Input: part model. Units: mm. Frame: model coordinates. A direction names the side the tool comes from. Give positions to 0.01 mm unless a question says otherwise; leave off trailing zeros. Loops run counter-clockwise (first coordinate to the right, second up) from the corner with the lowest first, then second, coordinate; pieces in that order, holes last. Notation, with made-up numbers: M 8.25,-18.5 L 44.25,-18.5 A6 cw 44.25,-12.5 Z; hole C 7.25,16.25 d2. An arc over 180 degrees is marked long. Use a Markdown table: item, result. Add a question column.
Autodesk Inventor part; units mm, degrees
ref_plane "YZ Plane" through (0, 0, 0) normal (1, 0, 0) x (0, 1, 0)
ref_plane "XZ Plane" through (0, 0, 0) normal (0, 1, 0) x (-1, 0, 0)
ref_plane "XY Plane" through (0, 0, 0) normal (0, 0, 1) x (1, 0, 0)
sketch "Sketch1" plane through (0, 0, 0) normal (0, 0, 1) x (1, 0, 0)
  line L0 (0, 0) -> (55, 0)
  line L1 (55, 0) -> (55, 55)
  line L2 (55, 55) -> (0, 55)
  line L3 (0, 55) -> (0, 0)
  dimension "d0" = 55
  dimension "d1" = 55
extrude "Extrusion1" add sketch "Sketch1" along normal blind 80
sketch "Sketch2" plane through (0, 0, 80) normal (0, 0, 1) x (1, 0, 0)
  line L0 (55, 0) -> (55, 55)
  line L1 (55, 55) -> (0, 55)
  line L2 (0, 55) -> (0, 0)
  line L3 (0, 0) -> (55, 0)
  circle A0 centre (27.5, 27.5) radius 20
  circle A1 centre (27.5, 27.5) radius 4
  dimension "d7" = 27.5
  dimension "d8" = 27.5
  dimension "d9" = 40
  dimension "d10" = 8
extrude "Extrusion2" add sketch "Sketch2" along normal blind 2 contours A0
sketch "Sketch3" plane through (27.5, 27.5, 80) normal (0, 0, 1) x (1, 0, 0)
  circle A0 centre (0, 0) radius 4
  point P0 (-27.5, -27.5)
extrude "Extrusion3" add sketch "Sketch3" along normal blind 30
chamfer "Chamfer1" distance 10 angle 45 4 edges at (0, 55, 40) (0, 0, 40) (55, 0, 40) (55, 55, 40)
sketch "Sketch4" plane through (0, 0, 80) normal (0, 0, 1) x (1, 0, 0)
  line L0 (45, 55) -> (55, 45)
  line L1 (45, 55) -> (10, 55)
  line L2 (0, 45) -> (10, 55)
  line L3 (0, 45) -> (0, 10)
  line L4 (10, 0) -> (0, 10)
  line L5 (10, 0) -> (45, 0)
  line L6 (55, 10) -> (45, 0)
  line L7 (55, 10) -> (55, 45)
  circle A0 centre (27.5, 27.5) radius 20
  line L8 (10, 55) -> (0, 55)
  line L9 (0, 55) -> (0, 45)
  line L10 (0, 10) -> (0, 0)
  line L11 (0, 0) -> (10, 0)
  line L12 (45, 0) -> (55, 0)
  line L13 (55, 0) -> (55, 10)
  line L14 (55, 45) -> (55, 55)
  line L15 (45, 55) -> (55, 55)
extrude "Extrusion4" add sketch "Sketch4" against normal blind 5 contours L15 L14 L0 | L2 L9 L8 | L13 L12 L6 | L4 L11 L10
sketch "Sketch5" plane through (0, 0, 80) normal (0, 0, 1) x (1, 0, 0)
  line L0 (0, 45) -> (10, 55)
  circle A0 centre (4, 51) radius 3
  line L1 (55, 55) -> (0, 55)
  line L2 (0, 55) -> (0, 0)
  circle A1 centre (4, 4) radius 3
  circle A2 centre (51, 4) radius 3
  circle A3 centre (51, 51) radius 3
  line L3 (0, 0) -> (55, 0)
  line L4 (55, 0) -> (55, 55)
  dimension "d20" = 4
  dimension "d21" = 4
  dimension "d22" = 6
  dimension "d23" = 4
  dimension "d24" = 4
  dimension "d25" = 4
  dimension "d26" = 4
  dimension "d27" = 4
  dimension "d28" = 4
extrude "Extrusion5" cut sketch "Sketch5" against normal through all contours A0 L0 | L0 A0 | A1 | A2 | A3
equation "\"d7\" = 0.5 * d1"
equation "\"d8\" = 0.5 * d0"
properties part number "stepper motor base" material "Aluminum"
1) Ray query, line 1 (Y direction, x = 4, z = 54); line 2 (Z direction, x = 38, y = 29); line 3 (Z direction, x = 7, y = 21). Return the intervals inside material, ascending. Write a range as [from, to].
2) Section query C-C, the plane z = 66. Return the cut outline in (x, y).
3) Section query D-D, the plane y = 38. Return the cut outline in (x, z), and give its area (3 significant figures).
4) Reachability of faces 1 (the flat face through (47, 53, 37)), 2 (the flat face through (2, 8, 38)), 3 (the cylindrical face through (24.55, 24.8, 95.8)), 4 (the flat face through (53, 1, 75)) from +Z, -Z, +X, -X, +Y, -Y: full face, straight path, thin tool, end or side. Return the list, or none.
5) Section query A-A, the plane x = 27.5. Return the cut outline in (y, z), and give its area (3 significant figures).
6) Contact query for flat-ended pins moving along their axis: P1, Ø2, axis at x = 32, z = 84.5, coming from the -Y side; P2, Ø9.5, axis at x = 51, y = 51, coming from the +Z side. Output: stop coordinate, or through.
Entries:
| question | item | result |
|---|---|---|
| 1 | line 1 | y = [7, 48] |
| 1 | line 2 | z = [0, 82] |
| 1 | line 3 | z = [0, 80] |
| 2 | outline | M 0,10 L 3.13,6.87 A3 cw 6.87,3.13 L 10,0 L 45,0 L 48.13,3.13 A3 cw 51.87,6.87 L 55,10 L 55,45 L 51.87,48.13 A3 cw 48.13,51.87 L 45,55 L 10,55 L 6.87,51.87 A3 cw 3.13,48.13 L 0,45 Z |
| 3 | outline | M 0,0 L 55,0 L 55,80 L 44.52,80 L 44.52,82 L 10.48,82 L 10.48,80 L 0,80 Z |
| 3 | area | 4,470 mm² |
| 4 | face 1 | -Z, +X, +Y |
| 4 | face 2 | -Z, -X, -Y |
| 4 | face 3 | +Z |
| 4 | face 4 | -Z, +X, -Y |
| 5 | outline | M 0,0 L 55,0 L 55,80 L 47.5,80 L 47.5,82 L 31.5,82 L 31.5,110 L 23.5,110 L 23.5,82 L 7.5,82 L 7.5,80 L 0,80 Z |
| 5 | area | 4,700 mm² |
| 6 | P1 | stops at y = 25.56 |
| 6 | P2 | stops at z = 80 |
